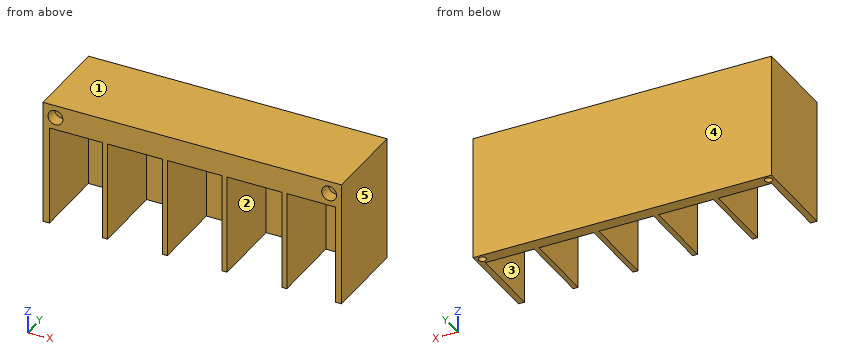
from build123d import *

# Parameters (mm, degrees)
SKETCH1_W           = 120
SKETCH1_H           = 50
BOSS_EXTRUDE1_DEPTH = 15
SKETCH2_W           = 24
SKETCH2_H           = 10
SKETCH2_W_2         = 2
SKETCH2_H_2         = 15
SKETCH2_W_3         = 1.99832088
BOSS_EXTRUDE2_DEPTH = 20
CUT_EXTRUDE1_DEPTH  = 10
SKETCH4_W           = 2
SKETCH4_H           = 30
SKETCH4_W_2         = 1.99832088
BOSS_EXTRUDE4_DEPTH = 40
SKETCH5_W           = 74
SKETCH5_H           = 15
CUT_EXTRUDE2_DEPTH  = 30
SKETCH6_R           = 3
CUT_EXTRUDE3_DEPTH  = 5
SKETCH7_W           = 2.440051729
SKETCH7_H           = 30
BOSS_EXTRUDE5_DEPTH = 40
SKETCH8_W           = 2.614904652
SKETCH8_H           = 30
BOSS_EXTRUDE6_DEPTH = 40
SKETCH9_R           = 1.5
CUT_EXTRUDE4_DEPTH  = 5


with BuildPart() as part:
    # Sketch1 → Boss-Extrude1 (new body)
    with BuildSketch(Plane(origin=(0, 0, 0), x_dir=(1, 0, 0), z_dir=(0, 1, 0))):
        with Locations((5.008183306, 25)):
            Rectangle(SKETCH1_W, SKETCH1_H)
    extrude(amount=BOSS_EXTRUDE1_DEPTH)

    # Sketch2 → Boss-Extrude2 (add)
    with BuildSketch(Plane.XZ):
        Polygon((-30.991816694, 0), (-30.991816694, -10), (-28.991816694, -10), (-6.991816694, -10), (-6.991816694, 0), align=None)
        with Locations((-42.991816694, -5)):
            Rectangle(SKETCH2_W, SKETCH2_H)
        with Locations((-29.991816694, -17.5)):
            Rectangle(SKETCH2_W_2, SKETCH2_H_2)
        with Locations((-5.992656254, -17.5)):
            Rectangle(SKETCH2_W_3, SKETCH2_H_2)
        Polygon((-6.991816694, 0), (-6.991816694, -10), (-4.993495814, -10), (17.008183306, -10), (17.008183306, 0), align=None)
        Polygon((41.008183306, 0), (17.008183306, 0), (17.008183306, -10), (19.008183306, -10), (41.008183306, -10), align=None)
        with Locations((18.008183306, -17.5)):
            Rectangle(SKETCH2_W_2, SKETCH2_H_2)
        Polygon((65.008183306, 0), (41.008183306, 0), (41.008183306, -10), (43.008183306, -10), (65.008183306, -10), align=None)
        with Locations((42.008183306, -17.5)):
            Rectangle(SKETCH2_W_2, SKETCH2_H_2)
    extrude(amount=BOSS_EXTRUDE2_DEPTH)

    # Sketch3 → Cut-Extrude1 (cut)
    with BuildSketch(Plane.XZ):
        Polygon((-54.991816694, -10), (-30.991816694, -10), (-30.991816694, -25), (-28.991816694, -25), (-28.991816694, -10), (-6.991816694, -10), (-6.991816694, -25), (-4.993495814, -25), (-4.993495814, -10), (17.008183306, -10), (17.008183306, -25), (19.008183306, -25), (19.008183306, -10), (41.008183306, -10), (41.008183306, -25), (43.008183306, -25), (43.008183306, -10), (65.008183306, -10), (65.008183306, -50), (-54.991816694, -50), align=None)
    extrude(amount=-CUT_EXTRUDE1_DEPTH, mode=Mode.SUBTRACT)

    # Sketch4 → Boss-Extrude4 (add)
    with BuildSketch(Plane(origin=(0, 0, -25), x_dir=(-1, 0, 0), z_dir=(0, 0, -1))):
        with Locations((29.991816694, -5)):
            Rectangle(SKETCH4_W, SKETCH4_H)
        with Locations((5.992656254, -5)):
            Rectangle(SKETCH4_W_2, SKETCH4_H)
        with Locations((-18.008183306, -5)):
            Rectangle(SKETCH4_W, SKETCH4_H)
        with Locations((-42.008183306, -5)):
            Rectangle(SKETCH4_W, SKETCH4_H)
    extrude(amount=BOSS_EXTRUDE4_DEPTH)

    # Sketch5 → Cut-Extrude2 (cut)
    with BuildSketch(Plane(origin=(0, 10, 0), x_dir=(1, 0, 0), z_dir=(0, 1, 0))):
        with Locations((6.008183306, 57.5)):
            Rectangle(SKETCH5_W, SKETCH5_H)
    extrude(amount=-CUT_EXTRUDE2_DEPTH, mode=Mode.SUBTRACT)

    # Sketch6 → Cut-Extrude3 (cut)
    with BuildSketch(Plane.XZ.offset(20)):
        with Locations(Location((-49.991816694, -5, 0), (0, 0, 270))):
            Circle(SKETCH6_R)
        with Locations(Location((60.008183306, -5, 0), (0, 0, 270))):
            Circle(SKETCH6_R)
    extrude(amount=-CUT_EXTRUDE3_DEPTH, mode=Mode.SUBTRACT)

    # Sketch7 → Boss-Extrude5 (add)
    with BuildSketch(Plane(origin=(0, 0, -10), x_dir=(-1, 0, 0), z_dir=(0, 0, -1))):
        with Locations((-63.788157442, -5)):
            Rectangle(SKETCH7_W, SKETCH7_H)
    extrude(amount=BOSS_EXTRUDE5_DEPTH)

    # Sketch8 → Boss-Extrude6 (add)
    with BuildSketch(Plane(origin=(0, 0, -10), x_dir=(-1, 0, 0), z_dir=(0, 0, -1))):
        with Locations((53.684364368, -5)):
            Rectangle(SKETCH8_W, SKETCH8_H)
    extrude(amount=BOSS_EXTRUDE6_DEPTH)

    # Sketch9 → Cut-Extrude4 (cut)
    with BuildSketch(Plane(origin=(0, 0, -50), x_dir=(-1, 0, 0), z_dir=(0, 0, -1))):
        with Locations((-62.508183306, 12.5)):
            Circle(SKETCH9_R)
        with Locations((52.491816694, 12.5)):
            Circle(SKETCH9_R)
    extrude(amount=-CUT_EXTRUDE4_DEPTH, mode=Mode.SUBTRACT)


solid = part.part
Work out the finished part from the listing and answer in its coordinate system (mm). Face numbers are marked on the shaded views. A direction names the side the tool comes from. Round coordinates to 2 decimals unless told otherwise and drop trailing zeros. Write each loop counter-clockwise with the first axis right and the second up, starting at its lowest first coordinate (ties: lowest second). Pieces come first, ordered by that corner, then holes. Notation, with made-up numbers: M -33,-18 L -17,-18 A21 cw -17,3 Z; hole C 83.25,63.25 d1. An arc over 180 degrees is marked long. Use a Markdown table: item, result.
1) The part is cut by section C-C on x = 29. Give the vertices of the cut face in (y, z), plus the area to 3 significant figures.
Taken from the geometry:
| item | result |
|---|---|
| outline | M -20,-10 L 10,-10 L 10,-50 L 15,-50 L 15,0 L -20,0 Z |
| area | 550 mm2 |
2) Flat-ended cylindrical pins translate along their axes: pin 1 (1.5 mm diameter, centred on x = 11, z = -32, fed in from -Y); pin 2 (6.5 mm diameter, centred on x = 31.5, y = -2, fed in from -Z); pin 3 (1.8 mm diameter, centred on x = 60, z = -4, fed in from -Y). Find the tip coordinate at first contact, or state that the pin passes through.
Taken from the geometry:
| item | result |
|---|---|
| pin 1 | stops at y = 10 |
| pin 2 | stops at z = -10 |
| pin 3 | stops at y = -15 |
3) The part is cut by section D-D on y = -9. Give the vertices of the cut face in (x, z).
Taken from the geometry:
| item | result |
|---|---|
| outline | M -54.99,-50 L -52.38,-50 L -52.38,-10 L -30.99,-10 L -30.99,-50 L -28.99,-50 L -28.99,-10 L -6.99,-10 L -6.99,-50 L -4.99,-50 L -4.99,-10 L 17.01,-10 L 17.01,-50 L 19.01,-50 L 19.01,-10 L 41.01,-10 L 41.01,-50 L 43.01,-50 L 43.01,-10 L 62.57,-10 L 62.57,-50 L 65.01,-50 L 65.01,0 L -54.99,0 Z |
4) The part is cut by section B-B on y = -16.5. Give the vertices of the cut face in (x, z).
Taken from the geometry:
| item | result |
|---|---|
| outline | M -54.99,-50 L -52.38,-50 L -52.38,-10 L -30.99,-10 L -30.99,-50 L -28.99,-50 L -28.99,-10 L -6.99,-10 L -6.99,-50 L -4.99,-50 L -4.99,-10 L 17.01,-10 L 17.01,-50 L 19.01,-50 L 19.01,-10 L 41.01,-10 L 41.01,-50 L 43.01,-50 L 43.01,-10 L 62.57,-10 L 62.57,-50 L 65.01,-50 L 65.01,0 L -54.99,0 Z; hole C -49.99,-5 d6; hole C 60.01,-5 d6 |
5) The part is cut by section A-A on z = -20. Give the vertices of the cut face in (x, y).
Taken from the geometry:
| item | result |
|---|---|
| outline | M -54.99,-20 L -52.38,-20 L -52.38,10 L -30.99,10 L -30.99,-20 L -28.99,-20 L -28.99,10 L -6.99,10 L -6.99,-20 L -4.99,-20 L -4.99,10 L 17.01,10 L 17.01,-20 L 19.01,-20 L 19.01,10 L 41.01,10 L 41.01,-20 L 43.01,-20 L 43.01,10 L 62.57,10 L 62.57,-20 L 65.01,-20 L 65.01,15 L -54.99,15 Z |
6) Which of the six approach directions +Z, -Z, +X, -X, +Y, -Y give full straight-line access (tool end or side, diameter ignored) to the marked faces 1 and 2?
Taken from the geometry:
| item | result |
|---|---|
| face 1 | +Z, +X, -X, +Y, -Y |
| face 2 | -Z, -Y |
7) Determine the mould class of the marked faces 3, 4 and 5 for opening direction X: pulls with the +X half, pulls with the -X half, needs draft (parallel to the pull), parting line crosses it, or undercut.
Taken from the geometry:
| item | result |
|---|---|
| face 3 | undercut |
| face 4 | needs draft |
| face 5 | pulls with the +X half |
8) Consider line 1 (X direction, y = -4, z = -20); line 2 (X direction, y = -17.95, z = -5); line 3 (Z direction, x = 24, y = -16). Determine where each line is inside the solid, lowest interval first. Write a range as [from, to].
Taken from the geometry:
| item | result |
|---|---|
| line 1 | x = [-54.99, -52.38], [-30.99, -28.99], [-6.99, -4.99], [17.01, 19.01], [41.01, 43.01], [62.57, 65.01] |
| line 2 | x = [-54.99, -52.99], [-46.99, 57.01], [63.01, 65.01] |
| line 3 | z = [-10, 0] |
